Design review of the part built by this model. Coordinates are the model's own, in mm. A direction names the side the tool comes from. Give positions to 0.01 mm unless a question says otherwise; leave off trailing zeros. Order: outer loops, then holes, each group sorted by start corner. A loop starts at its lowest first (then second) coordinate and runs counter-clockwise, first axis right, second up. Notation, with made-up numbers: (70, -34) -> (97, -34) arc R21 cw to (97, -24) -> close; hole circle Ø2 at (69, -36.5). An arc over 180 degrees is marked (long way). Answer in a Markdown table with one row per item. Add a question column.
```python
from build123d import *


with BuildPart() as part:
    # Schizzo2 → Rivoluzione2 (revolve)
    with BuildSketch(Plane(origin=(0, 0, 0), x_dir=(0, 0, -1), z_dir=(1, 0, 0)), mode=Mode.PRIVATE) as rivoluzione2_sk:
        Polygon((0, 0), (0, 3), (8.5, 3), (8.5, 4), (14, 4), (14, 6), (24, 6), (24, 8), (575, 8), (575, 6), (584.5, 6), (584.5, 4), (613.5, 4), (613.5, 3), (622, 3), (622, 0), align=None)
    revolve(rivoluzione2_sk.sketch.rotate(Axis((0, 0, 0), (0, 0, -1)), 90), axis=Axis((0, 0, 0), (0, 0, -1)))


solid = part.part
```
1) Add section C-C, the plane z = -174. Write out the cut boundary in (x, y), and give its area (3 significant figures).
2) For L1, parallel to Y at x = 0.5, z = -189; L2, parallel to Z at x = 3.5, y = 2.25; L3, parallel to X at y = -0.25, z = -291, list the stretches that pass through material, from the lowest coordinate up.
3) Clearance check with flat-ended pins moving along their axes: P1, Ø1.5, axis at x = -0.5, z = -550, coming from the +Y side; P2, Ø1.5, axis at y = 1.5, z = -75, coming from the +X side; P3, Ø1.5, axis at y = 1, z = -293.5, coming from the -X side; P4, Ø1, axis at y = 2.5, z = -163, coming from the -X side. State where each tip first meets the part, or that it passes through.
4) Add section A-A, the plane x = 0. Write out the cut boundary in (y, z), and give its area (3 significant figures).
5) Machinability: for faces 1 (the face through (1.42, 3.92, -14)), 2 (the face through (-2, -6, -575)), 3 (the face through (-1.73, 7.81, -303.36)), which of the approach directions +Z, -Z, +X, -X, +Y, -Y give a long, thin tool a straight path to every point of the face, cutting with its end or side? Answer none if there is none.
Verdict:
| question | item | result |
|---|---|---|
| 1 | outline | circle Ø16 at (0, 0) |
| 1 | area | 201 mm2 |
| 2 | L1 | y = -7.98 to 7.98 |
| 2 | L2 | z = -584.5 to -14 |
| 2 | L3 | x = -8 to 8 |
| 3 | P1 | stops at y = 8 |
| 3 | P2 | stops at x = 7.96 |
| 3 | P3 | stops at x = -8 |
| 3 | P4 | stops at x = -7.75 |
| 4 | outline | (-8, -575) -> (-6, -575) -> (-6, -584.5) -> (-4, -584.5) -> (-4, -613.5) -> (-3, -613.5) -> (-3, -622) -> (3, -622) -> (3, -613.5) -> (4, -613.5) -> (4, -584.5) -> (6, -584.5) -> (6, -575) -> (8, -575) -> (8, -24) -> (6, -24) -> (6, -14) -> (4, -14) -> (4, -8.5) -> (3, -8.5) -> (3, 0) -> (-3, 0) -> (-3, -8.5) -> (-4, -8.5) -> (-4, -14) -> (-6, -14) -> (-6, -24) -> (-8, -24) -> close |
| 4 | area | 9,430 mm2 |
| 5 | face 1 | +Z |
| 5 | face 2 | -Z |
| 5 | face 3 | +Z, -Z |
